from build123d import *

# Parameters (mm, degrees)
SKETCH1_R           = 53
SKETCH1_R_2         = 36.5
BOSS_EXTRUDE1_DEPTH = 20
SKETCH2_R           = 43.25
LED_RING_DEPTH      = 3
SKETCH3_R           = 40.1
SPINDLE_DEPTH       = 12
SKETCH4_R           = 4.5
LASERS_DEPTH        = 21


with BuildPart() as part:
    # Sketch1 → Boss-Extrude1 (new body)
    with BuildSketch(Plane(origin=(0, 0, 0), x_dir=(1, 0, 0), z_dir=(0, 1, 0))):
        Circle(SKETCH1_R)
        Circle(SKETCH1_R_2, mode=Mode.SUBTRACT)
    extrude(amount=BOSS_EXTRUDE1_DEPTH)

    # Sketch2 → LED-ring (cut)
    with BuildSketch(Plane(origin=(0, 20, 0), x_dir=(1, 0, 0), z_dir=(0, 1, 0))):
        Circle(SKETCH2_R)
    extrude(amount=-LED_RING_DEPTH, mode=Mode.SUBTRACT)

    # Sketch3 → spindle (cut)
    with BuildSketch(Plane.XZ):
        Circle(SKETCH3_R)
    extrude(amount=-SPINDLE_DEPTH, mode=Mode.SUBTRACT)

    # Sketch4 → lasers (cut, through all)
    with BuildSketch(Plane(origin=(0, 20, 0), x_dir=(1, 0, 0), z_dir=(0, 1, 0))):
        with Locations((0, 48)):
            Circle(SKETCH4_R)
        with Locations((48, 0)):
            Circle(SKETCH4_R)
    extrude(amount=-LASERS_DEPTH, mode=Mode.SUBTRACT)


solid = part.part
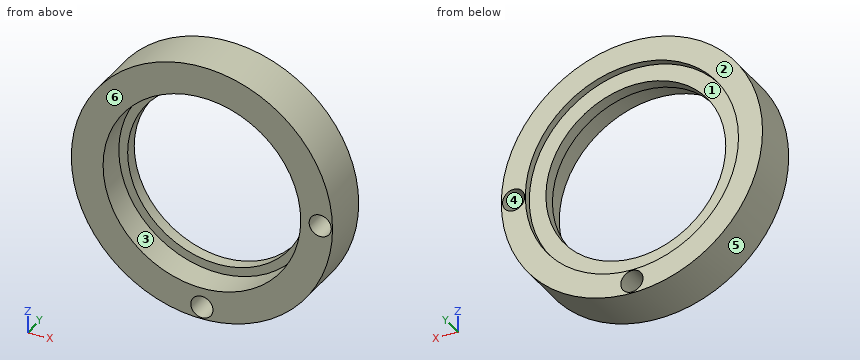
Source: CAD feature listing. Evaluate the final solid. Frame: model axes, mm. Face numbers are marked on the shaded views. A direction names the side the tool comes from. Round coordinates to 2 decimals unless told otherwise and drop trailing zeros. Loops run counter-clockwise (first coordinate to the right, second up) from the corner with the lowest first, then second, coordinate; pieces in that order, holes last.
Q1. First-contact query: P1, Ø1.5, axis at y = 6.5, z = 9, coming from the -X side; P2, Ø4, axis at y = 13.5, z = 9.5, coming from the +X side; P3, Ø5, axis at y = 16.5, z = 23, coming from the -X side. Flat tips, straight axial feed; report the tip coordinate or a pass-through.
Q2. Ray query, line 1 (Z direction, x = 0, y = 14.7); line 2 (Z direction, x = 0, y = 8.5); line 3 (X direction, y = 13.5, z = -17). Return the intervals inside material, ascending.
Q3. Section B-B, the plane z = -48. Return loops of the section in (x, y).
Q4. Mould query, pull axis Z, two halves, no side actions, for the marked faces 3, 4, 5 and 6. Classes: pulls with the +Z half, pulls with the -Z half, needs draft (parallel to the pull), parting line crosses it, or undercut.
Q5. Section D-D, the plane y = 14.75. Return loops of the section in (x, z).
Q6. Section A-A, the plane x = 0. Return loops of the section in (y, z), plus the area to 3 significant figures.
Q7. Access query for the marked faces 1 and 2. Directions: +Z, -Z, +X, -X, +Y, -Y. A direction counts if a zero-diameter tool reaches every point of the face in a straight line with its end or side. Return the directions, or none.
Q8. Section C-C, the plane x = 48. Return loops of the section in (y, z), plus the area to 3 significant figures.
Solutions:
1. P1: stops at x = -52.35
1. P2: stops at x = 52.47
1. P3: stops at x = -48.87
2. line 1: z = -53 to -52.5, -43.5 to -36.5, 36.5 to 53
2. line 2: z = -53 to -52.5, -43.5 to -40.1, 40.1 to 53
2. line 3: x = -50.2 to -32.3, 32.3 to 50.2
3. outline: (-22.47, 0) - (-4.5, 0) - (-4.5, 20) - (-22.47, 20) - close; (4.5, 0) - (22.47, 0) - (22.47, 20) - (4.5, 20) - close
4. face 3: undercut
4. face 4: undercut
4. face 5: parting line crosses it
4. face 6: needs draft
5. outline: circle Ø106 at (0, 0); hole circle Ø73 at (0, 0); hole circle Ø9 at (0, -48); hole circle Ø9 at (48, 0)
6. outline: (0, -53) - (20, -53) - (20, -52.5) - (0, -52.5) - close; (0, -43.5) - (20, -43.5) - (20, -43.25) - (17, -43.25) - (17, -36.5) - (12, -36.5) - (12, -40.1) - (0, -40.1) - close; (0, 40.1) - (12, 40.1) - (12, 36.5) - (17, 36.5) - (17, 43.25) - (20, 43.25) - (20, 53) - (0, 53) - close
6. area: 353 mm2
7. face 1: +Y
7. face 2: +Z, -Z, +X, -X, +Y
8. outline: (0, -22.47) - (20, -22.47) - (20, -4.5) - (0, -4.5) - close; (0, 4.5) - (20, 4.5) - (20, 22.47) - (0, 22.47) - close
8. area: 719 mm2
